Verification items for the finished model (mm, model axes). Coordinates: 2 decimals unless noted, no trailing zeros. Write each loop counter-clockwise with the first axis right and the second up, starting at its lowest first coordinate (ties: lowest second). Pieces come first, ordered by that corner, then holes. Notation, with made-up numbers: (-26, 17) -> (22, 17) arc R32 ccw to (22, 43) -> close; hole circle Ø5 at (19, 11). An arc over 180 degrees is marked (long way). Write item = value, one per line. Start each with the question number.
(1) Material ranges on probe 1 along X at (y, z) = (13, 0); probe 2 along Z at (x, y) = (16, 7); probe 3 along X at (y, z) = (16.25, 6.5), recorded low to high. Write a range as [from, to].
(2) Mould release check, pull along Z, two halves, no side actions. Record for faces 1 (the face through (27.3, 0, -4.7)), 2 (the face through (30.736, 8.881, -4.036)), 3 (the face through (-26.36, 8.88, -5.85)): released by +Z, released by -Z, zero draft, split by the parting line, or undercut.
(3) Gauge pin test, flat ends, axial feed: pin 1 Ø8 at (y, z) = (4, 13.5) entering from -X; pin 2 Ø2 at (x, y) = (3, 2) entering from +Z; pin 3 Ø10 at (y, z) = (16, 21) entering from -X. Record the tip position at first contact, or that the pin passes through.
(4) Section check A-A (z = 0). Record the cut outline in (x, y), plus the area to 3 significant figures.
(5) Section check C-C (y = 2.5). Record the cut outline in (x, z).
(6) Section check B-B (x = 0). Record the cut outline in (y, z), plus the area to 3 significant figures.
```python
from build123d import *

# Parameters (mm, degrees)
SCHIZZO1_R        = 31
SCHIZZO1_R_2      = 27
ESTRUSIONE1_DEPTH = 18
SMUSSO1_SIZE      = 0.5


with BuildPart() as part:
    # Schizzo1 → Estrusione1 (new body)
    with BuildSketch(Plane(origin=(0, 0, 0), x_dir=(1, 0, 0), z_dir=(0, 1, 0))):
        with Locations(Location((0, 0, 0), (0, 0, 270))):
            Circle(SCHIZZO1_R)
        with Locations(Location((0, 0, 0), (0, 0, 270))):
            Circle(SCHIZZO1_R_2, mode=Mode.SUBTRACT)
    extrude(amount=ESTRUSIONE1_DEPTH)

    # Smusso1
    smusso1_edges = [part.edges().sort_by_distance(p)[0] for p in [
        (0, 0, -31),
        (0, 18, -31),
        (0, 0, -27),
        (0, 18, -27),
    ]]
    chamfer(smusso1_edges, length=SMUSSO1_SIZE)


solid = part.part
```
Response:
q1.probe_1 = [-31, -27], [27, 31]
q1.probe_2 = [-26.55, -21.75], [21.75, 26.55]
q1.probe_3 = [-30.31, -26.21], [26.21, 30.31]
q2.face_1 = zero draft
q2.face_2 = split by the parting line
q2.face_3 = undercut
q3.pin_1 = -29.51
q3.pin_2 = 30.94
q3.pin_3 = -26.55
q4.outline = (-31, 0.5) -> (-30.5, 0) -> (-27.5, 0) -> (-27, 0.5) -> (-27, 17.5) -> (-27.5, 18) -> (-30.5, 18) -> (-31, 17.5) -> close; (27, 0.5) -> (27.5, 0) -> (30.5, 0) -> (31, 0.5) -> (31, 17.5) -> (30.5, 18) -> (27.5, 18) -> (27, 17.5) -> close
q4.area = 143 mm2
q5.outline = circle Ø62 at (0, 0); hole circle Ø54 at (0, 0)
q6.outline = (0, -30.5) -> (0.5, -31) -> (17.5, -31) -> (18, -30.5) -> (18, -27.5) -> (17.5, -27) -> (0.5, -27) -> (0, -27.5) -> close; (0, 27.5) -> (0.5, 27) -> (17.5, 27) -> (18, 27.5) -> (18, 30.5) -> (17.5, 31) -> (0.5, 31) -> (0, 30.5) -> close
q6.area = 143 mm2
